Autodesk Inventor part; units mm, degrees
ref_plane "YZ Plane" through (0, 0, 0) normal (1, 0, 0) x (0, 1, 0)
ref_plane "XZ Plane" through (0, 0, 0) normal (0, 1, 0) x (-1, 0, 0)
ref_plane "XY Plane" through (0, 0, 0) normal (0, 0, 1) x (1, 0, 0)
sketch "Sketch1" plane through (0, 0, 0) normal (0, 0, 1) x (1, 0, 0)
  line L0 (4.6821, 7.6658) -> (4.6821, 2.6658)
  line L1 (4.6821, 2.6658) -> (5.6821, 2.6658)
  line L2 (5.6821, 2.6658) -> (5.6821, -9.3342)
  line L3 (5.6821, -9.3342) -> (4.6821, -10.8342)
  line L4 (4.6821, -10.8342) -> (4.6821, -12.3342)
  line L5 (4.0821, -13.3342) -> (4.0821, -14.3342)
  line L6 (4.6821, -12.3342) -> (4.0821, -13.3342)
  line L7 (3.9321, -14.3342) -> (3.9321, -15.219)
  line L8 (3.6821, 7.6658) -> (3.6821, -15.2399)
  line L9 (4.0821, -14.3342) -> (3.9321, -14.3342)
  arc A0 (3.6821, -15.2399) -> (3.9321, -15.219) centre (3.7576, -14.6374) ccw
  line L10 (4.6821, 7.6658) -> (3.6821, 7.6658)
  point P0 (0, 0)
  dimension "d7" = 5
  dimension "d10" = 12
  dimension "d14" = 1
  dimension "d17" = 1.5
  dimension "d18" = 3
  dimension "d19" = 1
  dimension "d21" = 0.5
  dimension "d22" = 0.8
  dimension "d23" = 2
  dimension "d24" = 4
  dimension "d25" = 2
revolve "Revolution1" add sketch "Sketch1" angle 360 about axis through (3.6821, 7.6658, 0) along (0, -1, 0)
properties material "Nickel-Copper Alloy 400"
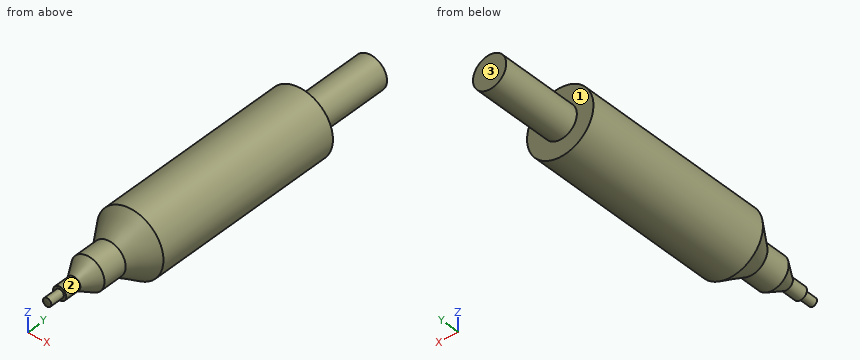
Can you work these out from the model? Positions are in its coordinate system, mm. Face numbers are marked on the shaded views. A direction names the side the tool comes from. Coordinates: 2 decimals unless noted, no trailing zeros. Order: outer loops, then holes, each group sorted by start corner. A loop starts at its lowest first (then second) coordinate and runs counter-clockwise, first axis right, second up. Notation, with made-up numbers: (46.5, 69.25) - (74.5, 69.25) arc R24 ccw to (74.5, 88.25) - close; hole circle Ø3 at (79, 11.5). An arc over 180 degrees is marked (long way). Answer in a Markdown table with one row per item.
1. For pin 1 (1.5 mm diameter, centred on y = 0.5, z = 1, fed in from +X); pin 2 (1.5 mm diameter, centred on x = 2, y = -6.5, fed in from -Z), each with a flat end and sliding along its axis, tell me the tip position at first contact or that it passes through.
Reply:
| item | result |
|---|---|
| pin 1 | stops at x = 5.67 |
| pin 2 | stops at z = -1.77 |
2. If I drill on line 1 along Y through (x, z) = (3.8, 0.3); line 2 along X through (y, z) = (-9.25, 0.1); line 3 along Y through (x, z) = (2.25, 0.1), over which ranges is the centre line in solid material (lowest first)?
Reply:
| item | result |
|---|---|
| line 1 | y = -14.33 to 7.67 |
| line 2 | x = 1.68 to 5.68 |
| line 3 | y = -10.18 to 2.67 |
3. Suppose I cut it at A-A (y = -3.75). Please give me the cut outline in (x, z).
Reply:
| item | result |
|---|---|
| outline | circle Ø4 at (3.68, 0) |
4. For the marked faces 1, 2 and 3, which set-ups out of +Z, -Z, +X, -X, +Y, -Y let a thin tool reach every point of the face, with its end or its side?
Reply:
| item | result |
|---|---|
| face 1 | +Y |
| face 2 | -Y |
| face 3 | +Z, -Z, +X, -X, +Y |
